```python
from build123d import *

# Parameters (mm, degrees)
CROQUIS1_R              = 1.58
CROQUIS1_R_2            = 14.25
SALIENTE_EXTRUIR1_DEPTH = 3
CROQUIS3_W              = 3
CROQUIS3_H              = 13.002457907
CROQUIS3_H_2            = 13.048194377
CROQUIS3_H_3            = 13.048194378
CORTAR_EXTRUIR1_DEPTH   = 3


with BuildPart() as part:
    # Croquis1 → Saliente-Extruir1 (new body)
    with BuildSketch(Plane.XY):
        with BuildLine():
            Line((-135.811178416, 31.660861846), (-65.873242367, 31.660861846))
            ThreePointArc((-65.873242367, 31.660861846), (-63.837291884, 32.094144685), (-62.154198363, 33.318899594))
            Line((-62.154198363, 33.318899594), (39.488020824, 146.429658271))
            ThreePointArc((39.488020824, 146.429658271), (43.775922453, 148.055230719), (47.585333219, 145.502393908))
            Line((47.585333219, 145.502393908), (132.043103592, -7.634273033))
            ThreePointArc((132.043103592, -7.634273033), (124.188821584, -34.806138154), (97.016956463, -26.951856146))
            Line((97.016956463, -26.951856146), (39.731279169, 76.917067288))
            ThreePointArc((39.731279169, 76.917067288), (35.921868403, 79.4699041), (31.633966774, 77.844331652))
            Line((31.633966774, 77.844331652), (-44.321252629, -6.681100406))
            ThreePointArc((-44.321252629, -6.681100406), (-46.00434615, -7.905855315), (-48.040296633, -8.339138154))
            Line((-48.040296633, -8.339138154), (-135.811178416, -8.339138154))
            ThreePointArc((-135.811178416, -8.339138154), (-155.811178416, 11.660861846), (-135.811178416, 31.660861846))
        make_face()
        with Locations((-135.811178416, 11.660861846)):
            Circle(CROQUIS1_R, mode=Mode.SUBTRACT)
        with Locations((-65.81121578, 11.5885363)):
            Circle(CROQUIS1_R, mode=Mode.SUBTRACT)
        with Locations((112.738617641, -14.044921514)):
            Circle(CROQUIS1_R_2, mode=Mode.SUBTRACT)
    extrude(amount=SALIENTE_EXTRUIR1_DEPTH)

    # Croquis3 → Cortar-Extruir1 (cut)
    with BuildSketch(Plane(origin=(98.018165522, 54.058873563, 0), x_dir=(0, 0, -1), z_dir=(0.875653678, 0.482939578, 0))):
        with Locations((-1.5, 79.927636726)):
            Rectangle(CROQUIS3_W, CROQUIS3_H)
        with Locations((-1.5, 49.42886568)):
            Rectangle(CROQUIS3_W, CROQUIS3_H_2)
        with Locations((-1.5, 18.952962868)):
            Rectangle(CROQUIS3_W, CROQUIS3_H_3)
    extrude(amount=-CORTAR_EXTRUIR1_DEPTH, mode=Mode.SUBTRACT)


solid = part.part
```
CAD build for the part. Positions are in the model's coordinates, mm. A direction names the side the tool comes from. Coordinates: 2 decimals unless noted, no trailing zeros. Loops run counter-clockwise (first coordinate to the right, second up) from the corner with the lowest first, then second, coordinate; pieces in that order, holes last. Notation, with made-up numbers: (31, -9) - (80, -9) arc R28 ccw to (80, 23) - close; hole circle Ø3 at (26, 71). An arc over 180 degrees is marked (long way). Return JSON: item names as keys, results as strings.
1. Band-saw the part on D-D (y = 68). Give the cut face in (x, z).
Result:
{"outline": "(-30.99, 0) - (22.79, 0) - (22.79, 3) - (-30.99, 3) - close; (44.65, 0) - (86.9, 0) - (86.9, 3) - (44.65, 3) - close"}
2. Band-saw the part on A-A (y = -23.5). Give the cut face in (x, z), and give its area (3 significant figures).
Result:
{"outline": "(95.11, 0) - (102.08, 0) - (102.08, 3) - (95.11, 3) - close; (123.4, 0) - (133.54, 0) - (133.54, 3) - (123.4, 3) - close", "area": "51.3 mm2"}
3. Band-saw the part on C-C (x = -109). Give the cut face in (y, z), and give its area (3 significant figures).
Result:
{"outline": "(-8.34, 0) - (31.66, 0) - (31.66, 3) - (-8.34, 3) - close", "area": "120 mm2"}
4. Mould opens along Y. For faces 3 (the flat face through (51.87, 137.73, 1.48)), 4 (the flat face through (86.19, 69.29, 1.52)), 5 (the flat face through (1, 49, 0)) say: released by +Y, released by -Y, zero draft, split by the parting line, or undercut.
Result:
{"face 3": "released by +Y", "face 4": "undercut", "face 5": "zero draft"}
5. 3-axis set-ups, long thin cutter, end or side, ignore diameter. For faces 1 (the flat face through (68.775, 24.256, 1.479)), 2 (the cylindrical face through (124.57, -34.59, 1.48)): which of +Z, -Z, +X, -X, +Y, -Y reach the whole face in a straight line?
Result:
{"face 1": "+Z, -Z, -Y", "face 2": "+Z, -Z"}
6. Drop flat-ended pins along their axis: pin 1 (5 mm diameter, centred on x = -135.81, y = 11.66, fed in from -Z); pin 2 (0.9 mm diameter, centred on x = -117.5, z = 2, fed in from +Y); pin 3 (0.9 mm diameter, centred on x = -111.5, z = 1.5, fed in from -Y). Give the stop position or say it passes through.
Result:
{"pin 1": "stops at z = 0", "pin 2": "stops at y = 31.66", "pin 3": "stops at y = -8.34"}
7. Band-saw the part on B-B (z = 1.25). Give the cut face in (x, y).
Result:
{"outline": "(-135.81, -8.34) - (-48.04, -8.34) arc R5 ccw to (-44.32, -6.68) - (31.63, 77.84) arc R5 cw to (39.73, 76.92) - (97.02, -26.95) arc R20 ccw to (132.04, -7.63) - (92.02, 64.94) - (89.39, 63.49) - (83.09, 74.92) - (85.71, 76.37) - (77.3, 91.63) - (74.67, 90.18) - (68.37, 101.61) - (71, 103.05) - (62.56, 118.35) - (59.93, 116.91) - (53.65, 128.29) - (56.28, 129.74) - (47.59, 145.5) arc R5 ccw to (39.49, 146.43) - (-62.15, 33.32) arc R5 cw to (-65.87, 31.66) - (-135.81, 31.66) arc R20 ccw to start; hole circle Ø3.16 at (-135.81, 11.66); hole circle Ø3.16 at (-65.81, 11.59); hole circle Ø28.5 at (112.74, -14.04)"}
8. Probe L1, parallel to X at y = 33.5, z = 2.75; L2, parallel to X at y = 49.5, z = 2.85; L3, parallel to Y at x = -86.5, z = 0.35. List the from-to ranges inside material, lowest first. Write a range as from..to.
Result:
{"L1": "x = -61.99..-8.21, 63.68..109.36", "L2": "x = -47.61..6.16, 54.85..100.53", "L3": "y = -8.34..31.66"}
